The listing builds one solid part. Answer for the finished solid, in the listing's coordinates (mm). Face numbers are marked on the shaded views. A direction names the side the tool comes from. Give positions to 0.01 mm unless a question says otherwise; leave off trailing zeros. Loops run counter-clockwise (first coordinate to the right, second up) from the corner with the lowest first, then second, coordinate; pieces in that order, holes last. Notation, with made-up numbers: (79.25, 62.25) -> (110.25, 62.25) arc R33 cw to (110.25, 97.25) -> close; hole circle Ø2 at (27.25, -22.5). An arc over 180 degrees is marked (long way). One line per question, with ' | ' between items. Start each with the question number.
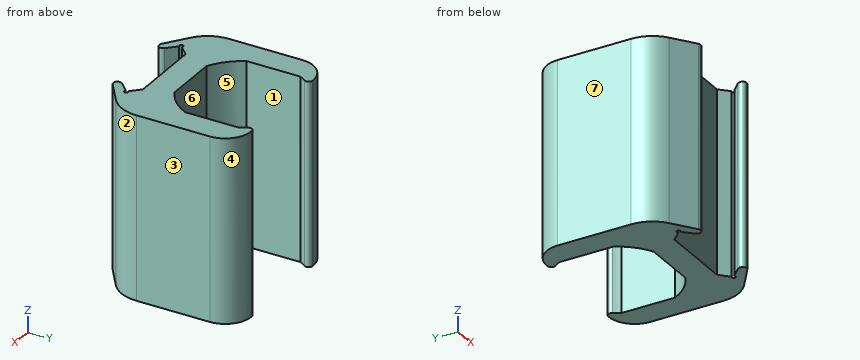
from build123d import *

# Parameters (mm, degrees)
F1_DEPTH = 44.45


with BuildPart() as f1:
    # F0 (on Top) → F1 (new body)
    with BuildSketch(Plane.XY):
        with BuildLine():
            Line((-10.949447, -21.236447), (-8.763, -19.05))
            Line((-8.763, -19.05), (8.763, -19.05))
            Line((8.763, -19.05), (10.949447, -21.236447))
            ThreePointArc((10.949447, -21.236447), (11.803, -21.59), (10.949447, -21.943553))
            Line((10.949447, -21.943553), (8.763, -24.13))
            ThreePointArc((8.763, -24.13), (8.711187, -25.48829), (10.061583, -25.643429))
            Line((10.061583, -25.643429), (15.41822, -21.714082))
            ThreePointArc((15.41822, -21.714082), (18.090248, -18.563741), (19.05, -14.545873))
            Line((19.05, -14.545873), (19.05, 3.272715))
            ThreePointArc((19.05, 3.272715), (17.190128, 7.762843), (12.7, 9.622715))
            Line((12.7, 9.622715), (12.533354, 9.622715))
            ThreePointArc((12.533354, 9.622715), (11.68973, 9.11243), (11.75002, 8.128327))
            ThreePointArc((11.75002, 8.128327), (12.250602, 7.352238), (12.7, 6.54543))
            Line((12.7, 6.54543), (12.7, -6.54543))
            ThreePointArc((12.7, -6.54543), (10.102788, -10.102788), (6.54543, -12.7))
            Line((6.54543, -12.7), (-6.54543, -12.7))
            ThreePointArc((-6.54543, -12.7), (-10.102788, -10.102788), (-12.7, -6.54543))
            Line((-12.7, -6.54543), (-12.7, 6.54543))
            ThreePointArc((-12.7, 6.54543), (-12.250602, 7.352238), (-11.75002, 8.128327))
            ThreePointArc((-11.75002, 8.128327), (-11.68973, 9.11243), (-12.533354, 9.622715))
            Line((-12.533354, 9.622715), (-12.7, 9.622715))
            ThreePointArc((-12.7, 9.622715), (-17.190128, 7.762843), (-19.05, 3.272715))
            Line((-19.05, 3.272715), (-19.05, -14.545873))
            ThreePointArc((-19.05, -14.545873), (-18.090248, -18.563741), (-15.41822, -21.714082))
            Line((-15.41822, -21.714082), (-10.061583, -25.643429))
            ThreePointArc((-10.061583, -25.643429), (-8.711187, -25.48829), (-8.763, -24.13))
            Line((-8.763, -24.13), (-10.949447, -21.943553))
            ThreePointArc((-10.949447, -21.943553), (-11.803, -21.59), (-10.949447, -21.236447))
        make_face()
    extrude(amount=F1_DEPTH)


solid = f1.part
1. The part is cut by section A-A (y = -2). Write down the section's boundary in (x, z), plus the area to 3 significant figures.
2. The part is cut by section C-C (x = 2). Write down the section's boundary in (y, z), plus the area to 3 significant figures.
3. For the marked faces 5, 6 and 7, determine the directions among +Z, -Z, +X, -X, +Y, -Y from which every point of the face is accessible in a straight line to the end or side of a thin tool.
4. Determine the mould class of the marked faces 1, 2, 3 and 4 for opening direction Y: released by +Y, released by -Y, zero draft, split by the parting line, or undercut.
5. Straight lines are drawn through the part: L1, parallel to X at y = 2, z = 5.5; L2, parallel to Y at x = 0, z = 2.5; L3, parallel to X at y = -21.59, z = 20. For each, find the intervals that lie inside material, in ascending order.
6. Each of these flat-tipped pins is pushed along its axis until it touches: pin 1 Ø12 at (x, z) = (5, 32) entering from -Y; pin 2 Ø4 at (x, z) = (-2.5, 14) entering from +Y; pin 3 Ø8 at (x, y) = (5.5, -8) entering from -Z. Where does it stop, or does it pass through?
7. The part is cut by section D-D (y = -8). Write down the section's boundary in (x, z), plus the area to 3 significant figures.
Check sheet entries:
1) outline: (-19.05, 0) -> (-12.7, 0) -> (-12.7, 44.45) -> (-19.05, 44.45) -> close; (12.7, 0) -> (19.05, 0) -> (19.05, 44.45) -> (12.7, 44.45) -> close | area: 565 mm^2
2) outline: (-19.05, 0) -> (-12.7, 0) -> (-12.7, 44.45) -> (-19.05, 44.45) -> close | area: 282 mm^2
3) face 5: +Z, -Z | face 6: +Z, -Z, +Y | face 7: +Z, -Z, -X, +Y, -Y
4) face 1: undercut | face 2: released by -Y | face 3: zero draft | face 4: released by +Y
5) L1: x = -19.05 to -12.7, 12.7 to 19.05 | L2: y = -19.05 to -12.7 | L3: x = -15.58 to -11.8, 11.8 to 15.58
6) pin 1: stops at y = -25.84 | pin 2: stops at y = -12.7 | pin 3: passes through
7) outline: (-19.05, 0) -> (-11.84, 0) -> (-11.84, 44.45) -> (-19.05, 44.45) -> close; (11.84, 0) -> (19.05, 0) -> (19.05, 44.45) -> (11.84, 44.45) -> close | area: 641 mm^2
